from build123d import *

# Parameters (mm, degrees)
SKETCH1_R                                     = 37.5
BOSS_EXTRUDE1_DEPTH                           = 6
TROU_POUR_TARAUDAGE_POUR_TROU_TARAUD_M8_D     = 6.8
TROU_POUR_TARAUDAGE_POUR_TROU_TARAUD_M8_DEPTH = 23
TROU_POUR_TARAUDAGE_POUR_TROU_TARAUD_M8_TIP   = 2.042926105
SKETCH6_R                                     = 14.5
BOSS_EXTRU_1_DEPTH                            = 6
SKETCH5_R                                     = 12.5
BOSS_EXTRU_2_DEPTH                            = 21.25
ESQUISSE11_R                                  = 7.5
BOSS_EXTRU_6_DEPTH                            = 20.5
TROU_POUR_TARAUDAGE_POUR_TROU_TARAUD_M6_D     = 5
TROU_POUR_TARAUDAGE_POUR_TROU_TARAUD_M6_DEPTH = 24
TROU_POUR_TARAUDAGE_POUR_TROU_TARAUD_M6_TIP   = 1.502151548
ENL_V_MAT_EXTRU_1_DEPTH                       = 34


with BuildPart() as part:
    # Sketch1 → Boss-Extrude1 (new body)
    with BuildSketch(Plane.XY):
        Circle(SKETCH1_R)
    extrude(amount=BOSS_EXTRUDE1_DEPTH)

    # Trou pour taraudage pour trou taraudé M81
    with Locations(Plane.XY.offset(6)):
        with Locations((-30, 0), (0, 30), (30, 0), (0, -30)):
            Hole(TROU_POUR_TARAUDAGE_POUR_TROU_TARAUD_M8_D / 2, depth=TROU_POUR_TARAUDAGE_POUR_TROU_TARAUD_M8_DEPTH)
            with Locations((0, 0, -(TROU_POUR_TARAUDAGE_POUR_TROU_TARAUD_M8_DEPTH + TROU_POUR_TARAUDAGE_POUR_TROU_TARAUD_M8_TIP / 2))):  # 118° drill point
                Cone(0, TROU_POUR_TARAUDAGE_POUR_TROU_TARAUD_M8_D / 2, TROU_POUR_TARAUDAGE_POUR_TROU_TARAUD_M8_TIP, mode=Mode.SUBTRACT)

    # Sketch6 → Boss.-Extru.1 (add)
    with BuildSketch(Plane(origin=(0, 0, 0), x_dir=(-1, 0, 0), z_dir=(0, 0, -1))):
        Circle(SKETCH6_R)
    extrude(amount=BOSS_EXTRU_1_DEPTH)

    # Sketch5 → Boss.-Extru.2 (add)
    with BuildSketch(Plane(origin=(0, 0, -6), x_dir=(-1, 0, 0), z_dir=(0, 0, -1))):
        Circle(SKETCH5_R)
    extrude(amount=BOSS_EXTRU_2_DEPTH)

    # Esquisse11 → Boss.-Extru.6 (add)
    with BuildSketch(Plane(origin=(0, 0, -27.25), x_dir=(-1, 0, 0), z_dir=(0, 0, -1))):
        Circle(ESQUISSE11_R)
    extrude(amount=BOSS_EXTRU_6_DEPTH)

    # Trou pour taraudage pour trou taraudé M61
    with Locations(Plane(origin=(0, 0, -47.75), x_dir=(-1, 0, 0), z_dir=(0, 0, -1))):
        with Locations((0, 0)):
            Hole(TROU_POUR_TARAUDAGE_POUR_TROU_TARAUD_M6_D / 2, depth=TROU_POUR_TARAUDAGE_POUR_TROU_TARAUD_M6_DEPTH)
            with Locations((0, 0, -(TROU_POUR_TARAUDAGE_POUR_TROU_TARAUD_M6_DEPTH + TROU_POUR_TARAUDAGE_POUR_TROU_TARAUD_M6_TIP / 2))):  # 118° drill point
                Cone(0, TROU_POUR_TARAUDAGE_POUR_TROU_TARAUD_M6_D / 2, TROU_POUR_TARAUDAGE_POUR_TROU_TARAUD_M6_TIP, mode=Mode.SUBTRACT)

    # Esquisse5 → Enlèv. mat.-Extru.1 (cut, through all)
    with BuildSketch(Plane(origin=(0, -4.5, 0), x_dir=(1, 0, 0), z_dir=(0, 1, 0))):
        with BuildLine():
            Line((2.5, 47.75), (2.5, 30.75))
            ThreePointArc((2.5, 30.75), (0, 28.25), (-2.5, 30.75))
            Line((-2.5, 30.75), (-2.5, 47.75))
            ThreePointArc((-2.5, 47.75), (0, 50.25), (2.5, 47.75))
        make_face()
    extrude(amount=-ENL_V_MAT_EXTRU_1_DEPTH, mode=Mode.SUBTRACT)


solid = part.part
Model file for the job. Use its own axes, mm. A direction names the side the tool comes from. Coordinates: 2 decimals unless noted, no trailing zeros. Order: outer loops, then holes, each group sorted by start corner. A loop starts at its lowest first (then second) coordinate and runs counter-clockwise, first axis right, second up. Notation, with made-up numbers: (-20.5, -22) -> (20.5, -22) arc R23 ccw to (20.5, -1) -> close; hole circle Ø2 at (35, 28). An arc over 180 degrees is marked (long way). Return JSON: item names as keys, results as strings. Group by question number.
Item 1: Pull direction X, two halves, no side cores. Call faces 4 (the cylindrical face through (0.44, -26.63, 2.96)), 5 (the cylindrical face through (-6.691, -12.864, -2.958)), 6 (the flat face through (0, -8, -27.25)): pulls with the +X half, pulls with the -X half, needs draft (parallel to the pull), parting line crosses it, or undercut.
Item 2: Wall check: line 1 along Y through (x, z) = (0, 2.65); line 2 along Y through (x, z) = (0, -29.75); line 3 along Z through (x, y) = (-7.5, 6). Give the ranges that are in metal, low to high. Write a range as [from, to].
Item 3: Saw through at B-B on z = -38. Write the cut outline in (x, y).
Item 4: Flat gauge pins, fed straight in: P1, Ø3, axis at x = 9.5, y = 28, coming from the -Z side; P2, Ø8, axis at x = 0, y = 0, coming from the -Z side; P3, Ø1.3, axis at y = -5.5, z = -42, coming from the +X side; P4, Ø2.5, axis at x = -1, z = -40.5, coming from the -Y side. Where does each tip first touch, or does it go through?
Item 5: Saw through at A-A on x = 30. Write the cut outline in (y, z).
Item 6: Saw through at C-C on y = -11.5. Write the cut outline in (x, z).
Item 7: Saw through at D-D on z = -11. Write the cut outline in (x, y).
Item 8: Tool access for faces 1 (the flat face through (2.5, -6, -39)), 2 (the flat face through (16, 1, 0)), 3 (the flat face through (2, 2, -47.75)): list every direction of +Z, -Z, +X, -X, +Y, -Y with a clear straight run to the whole face (end or side of a thin tool).
Values found:
{
 "1": {"face 4": "undercut", "face 5": "parting line crosses it", "face 6": "needs draft"},
 "2": {"line 1": "y = [-37.5, -33.4], [-26.6, 26.6], [33.4, 37.5]", "line 2": "y = [-4.5, -2.5], [2.5, 7.5]", "line 3": "z = [-27.25, 6]"},
 "3": {"outline": "(-2.5, -7.07) -> (-2.5, -4.5) -> (2.5, -4.5) -> (2.5, -7.07) arc R7.5 ccw (long way) to start; hole circle Ø5 at (0, 0)"},
 "4": {"P1": "stops at z = 0", "P2": "stops at z = -47.75", "P3": "stops at x = 5.72", "P4": "stops at y = -4.5"},
 "5": {"outline": "(-22.5, 0) -> (-3.4, 0) -> (-3.4, 6) -> (-22.5, 6) -> close; (3.4, 0) -> (22.5, 0) -> (22.5, 6) -> (3.4, 6) -> close"},
 "6": {"outline": "(-35.69, 0) -> (-8.83, 0) -> (-8.83, -6) -> (-4.9, -6) -> (-4.9, -27.25) -> (4.9, -27.25) -> (4.9, -6) -> (8.83, -6) -> (8.83, 0) -> (35.69, 0) -> (35.69, 6) -> (-35.69, 6) -> close"},
 "7": {"outline": "circle Ø25 at (0, 0)"},
 "8": {"face 1": "-Z, -Y", "face 2": "-Z", "face 3": "-Z, +X, -X, +Y, -Y"}
}
